```python
from build123d import *

# Parameters (mm, degrees)
BOSS_STRUCTURE_START                            = -40
BOSS_STRUCTURE_OUTLINE_W                        = 10
BOSS_STRUCTURE_OUTLINE_H                        = 70
BOSS_STRUCTURE_DEPTH                            = 80
SKETCH3_W                                       = 70
SKETCH3_H                                       = 5
BOSS_ATTACHE_AVANT_DEPTH                        = 12
SKETCH4_W                                       = 70
SKETCH4_H                                       = 5
BOSS_ATTACHE_ARRI_RE_DEPTH                      = 12
CBORE_FOR_6_PAN_HEAD_MACHINE_SCREW1_D           = 4.3053
CBORE_FOR_6_PAN_HEAD_MACHINE_SCREW1_CBORE_D     = 11.000000098
CBORE_FOR_6_PAN_HEAD_MACHINE_SCREW1_CBORE_DEPTH = 3.000000096
F_6_CLEARANCE_HOLE1_D                           = 4.3053
SKETCH10_W                                      = 12
SKETCH10_H                                      = 12
CUT_SUPPORT_LAT_DEPTH                           = 5
F_6_CLEARANCE_HOLE2_D                           = 4.3053
F_6_CLEARANCE_HOLE2_DEPTH                       = 10
BOARD_R                                         = 2
CUT_EXTRUDE2_DEPTH                              = 6.5


# Read off the part's stored shape, not the designer's step: Boss-Structure
with BuildPart() as part:
    # Boss-Structure outline → Boss-Structure (new body)
    with BuildSketch(Plane.YZ.offset(BOSS_STRUCTURE_START)):
        with Locations((-5, 0)):
            Rectangle(BOSS_STRUCTURE_OUTLINE_W, BOSS_STRUCTURE_OUTLINE_H)
    extrude(amount=BOSS_STRUCTURE_DEPTH)

    # Sketch3 → Boss-Attache avant (add)
    with BuildSketch(Plane.ZY.offset(40)):
        with Locations((0, -2.5)):
            Rectangle(SKETCH3_W, SKETCH3_H)
    extrude(amount=BOSS_ATTACHE_AVANT_DEPTH)

    # Sketch4 → Boss-Attache arrière (add)
    with BuildSketch(Plane(origin=(40, 0, 0), x_dir=(0, 0, -1), z_dir=(1, 0, 0))):
        with Locations((0, -7.5)):
            Rectangle(SKETCH4_W, SKETCH4_H)
    extrude(amount=BOSS_ATTACHE_ARRI_RE_DEPTH)

    # CBORE for #6 Pan Head Machine Screw1 (through all)
    with Locations(Plane(origin=(0, 0, 0), x_dir=(1, 0, 0), z_dir=(0, 1, 0))):
        with Locations((-46, 20), (-46, -20)):
            CounterBoreHole(CBORE_FOR_6_PAN_HEAD_MACHINE_SCREW1_D / 2, CBORE_FOR_6_PAN_HEAD_MACHINE_SCREW1_CBORE_D / 2, CBORE_FOR_6_PAN_HEAD_MACHINE_SCREW1_CBORE_DEPTH)

    # #6 Clearance Hole1 (through all)
    with Locations(Plane(origin=(0, -5, 0), x_dir=(1, 0, 0), z_dir=(0, 1, 0))):
        with Locations((46, 20), (46, -20)):
            Hole(F_6_CLEARANCE_HOLE1_D / 2)

    # Sketch10 → Cut-Support lat (cut)
    with BuildSketch(Plane.XZ.offset(10)):
        with Locations((29, 29)):
            Rectangle(SKETCH10_W, SKETCH10_H)
        with Locations((29, -29)):
            Rectangle(SKETCH10_W, SKETCH10_H)
    extrude(amount=-CUT_SUPPORT_LAT_DEPTH, mode=Mode.SUBTRACT)

    # #6 Clearance Hole2
    with Locations(Plane(origin=(0, 0, 0), x_dir=(1, 0, 0), z_dir=(0, 1, 0))):
        with Locations((-34, 29), (-34, -29), (29, -29), (29, 29)):
            Hole(F_6_CLEARANCE_HOLE2_D / 2, depth=F_6_CLEARANCE_HOLE2_DEPTH)

    # Board → Cut-Extrude2 (cut)
    with BuildSketch(Plane(origin=(0, 0, 0), x_dir=(1, 0, 0), z_dir=(0, 1, 0))):
        with Locations(Location((-12, 27.75, 0), (0, 0, 270))):
            Circle(BOARD_R)
        with Locations(Location((7, 27.75, 0), (0, 0, 270))):
            Circle(BOARD_R)
        with Locations(Location((-12, -27.75, 0), (0, 0, 270))):
            Circle(BOARD_R)
        with Locations(Location((7, -27.75, 0), (0, 0, 270))):
            Circle(BOARD_R)
        with Locations(Location((27, 2, 0), (0, 0, 270))):
            Circle(BOARD_R)
    extrude(amount=-CUT_EXTRUDE2_DEPTH, mode=Mode.SUBTRACT)


solid = part.part
```
Check sheet for the modelled part. Datum: model origin and axes. Units: mm. A direction names the side the tool comes from. Give positions to 0.01 mm unless a question says otherwise; leave off trailing zeros. Order: outer loops, then holes, each group sorted by start corner. A loop starts at its lowest first (then second) coordinate and runs counter-clockwise, first axis right, second up. Notation, with made-up numbers: M 77.5,22 L 136.5,22 A26 ccw 136.5,37 Z; hole C 67,14 d4. An arc over 180 degrees is marked long. Answer in a Markdown table with one row per item.
1) Access from +Z, -Z, +X, -X, +Y, -Y to the whole of each face (thin tool, end or side, straight path). Record for faces 3 (the cylindrical face through (-51.495, -1.479, 19.758)), 4 (the flat face through (35, -8, 29)), 5 (the flat face through (32, -5, -29)).
Filled sheet:
| item | result |
|---|---|
| face 3 | +Y |
| face 4 | +Z, -Y |
| face 5 | -Z, -Y |
2) Cross-section at C-C, the plane z = -2. Enter the section's corners in (x, y).
Filled sheet:
| item | result |
|---|---|
| outline | M -52,-5 L -40,-5 L -40,-10 L 52,-10 L 52,-5 L 40,-5 L 40,0 L 29,0 L 29,-6.5 L 25,-6.5 L 25,0 L -52,0 Z |
3) Thickness scan on L1, parallel to Z at x = -46, y = -1.5; L2, parallel to Z at x = -46, y = -3.45; L3, parallel to X at y = -6.05, z = 20. Record the ranges inside material, lowest first. Write a range as [from, to].
Filled sheet:
| item | result |
|---|---|
| L1 | z = [-35, -25.5], [-14.5, 14.5], [25.5, 35] |
| L2 | z = [-35, -22.15], [-17.85, 17.85], [22.15, 35] |
| L3 | x = [-40, 43.85], [48.15, 52] |
4) Cross-section at B-B, the plane z = 20. Enter the section's corners in (x, y).
Filled sheet:
| item | result |
|---|---|
| outline | M -52,-5 L -48.15,-5 L -48.15,-3 L -51.5,-3 L -51.5,0 L -52,0 Z; M -43.85,-5 L -40,-5 L -40,-10 L 43.85,-10 L 43.85,-5 L 40,-5 L 40,0 L -40.5,0 L -40.5,-3 L -43.85,-3 Z; M 48.15,-10 L 52,-10 L 52,-5 L 48.15,-5 Z |
5) Gauge pin test, flat ends, axial feed: P1, Ø4, axis at x = 30, y = -8.5, coming from the +Z side; P2, Ø10, axis at x = -46, z = -20, coming from the -Y side; P3, Ø3, axis at y = -8.5, z = -2.5, coming from the -X side; P4, Ø3.5, axis at x = -46, z = 20, coming from the -Y side. Record the tip position at first contact, or that the pin passes through.
Filled sheet:
| item | result |
|---|---|
| P1 | stops at z = 23 |
| P2 | stops at y = -5 |
| P3 | stops at x = -40 |
| P4 | passes through |
6) Cross-section at D-D, the plane x = -46. Enter the section's corners in (y, z).
Filled sheet:
| item | result |
|---|---|
| outline | M -5,-35 L 0,-35 L 0,-25.5 L -3,-25.5 L -3,-22.15 L -5,-22.15 Z; M -5,-17.85 L -3,-17.85 L -3,-14.5 L 0,-14.5 L 0,14.5 L -3,14.5 L -3,17.85 L -5,17.85 Z; M -5,22.15 L -3,22.15 L -3,25.5 L 0,25.5 L 0,35 L -5,35 Z |
7) Release check for a two-part mould opening along X. For faces 1 (the cylindrical face through (44.843, -7.535, -21.815)), 2 (the flat face through (46, -5, 0)) record: +X half, -X half, draft (parallel to the pull), parting line (faces both ways), or undercut.
Filled sheet:
| item | result |
|---|---|
| face 1 | undercut |
| face 2 | draft |
8) Cross-section at A-A, the plane x = -34. Enter the section's corners in (y, z), plus the area to 3 significant figures.
Filled sheet:
| item | result |
|---|---|
| outline | M -10,-35 L 0,-35 L 0,-31.15 L -10,-31.15 Z; M -10,-26.85 L 0,-26.85 L 0,26.85 L -10,26.85 Z; M -10,31.15 L 0,31.15 L 0,35 L -10,35 Z |
| area | 614 mm2 |
